Geometry check sheet. Reference: the model listing, model coordinates, mm. A direction names the side the tool comes from. Give positions to 0.01 mm unless a question says otherwise; leave off trailing zeros. Write each loop counter-clockwise with the first axis right and the second up, starting at its lowest first coordinate (ties: lowest second). Pieces come first, ordered by that corner, then holes. Notation, with made-up numbers: (57.25, 35) -> (81.25, 35) arc R7 cw to (81.25, 46) -> close; hole circle Ø7 at (-38.5, -3.75). An arc over 180 degrees is marked (long way). Write item = value, one per line. Start each with the question number.
1. Set-up check for faces 4 (the flat face through (25, 11, -15)), 5 (the flat face through (17, 23, -12)), 6 (the flat face through (3, 11, -15)), 7 (the cylindrical face through (14.07, 20.45, -12.5)): record each of +Z, -Z, +X, -X, +Y, -Y from which the full face is reachable in a straight line by a thin tool's end or side.
2. Cross-section at B-B, the plane x = 14. Record the cut outline in (y, z).
3. Cross-section at C-C, the plane z = -17. Record the cut outline in (x, y), plus the area to 3 significant figures.
4. Cross-section at A-A, the plane y = 11.5. Record the cut outline in (x, z), plus the area to 3 significant figures.
5. Thickness scan on line 1 along X through (y, z) = (19.8, -11); line 2 along Y through (x, z) = (14, -10.25); line 3 along X through (y, z) = (16.75, -1). Record the ranges inside material, lowest first.
6. Cross-section at D-D, the plane x = 8.75. Record the cut outline in (y, z), plus the area to 3 significant figures.
7. Depth check by flat-ended pin: P1, Ø10, axis at y = 8, z = -18.5, coming from the -X side; P2, Ø5, axis at y = 15, z = -13, coming from the +X side; P3, Ø1.5, axis at x = 27, y = 15, coming from the -Z side. Enter the tip coordinate at first touch or a pass-through.
8. Mould release check, pull along X, two halves, no side actions. Record for faces 1 (the cylindrical face through (12.483, 4.666, -11.339)), 2 (the flat face through (19, 6, -23)), 3 (the flat face through (0, 11, -4)): pulls with the +X half, pulls with the -X half, needs draft (parallel to the pull), parting line crosses it, or undercut.
```python
from build123d import *

# Parameters (mm, degrees)
BOSS_EXTRUDE1_DEPTH = 23
SKETCH2_R           = 7
CUT_EXTRUDE1_DEPTH  = 43.918527468
SKETCH3_R           = 1.5
CUT_EXTRUDE2_DEPTH  = 10
CHAMFER1_SIZE       = 0.5


with BuildPart() as part:
    # Sketch1 → Boss-Extrude1 (new body)
    with BuildSketch(Plane(origin=(0, 0, 0), x_dir=(1, 0, 0), z_dir=(0, 1, 0))):
        Polygon((0, 0), (28, 0), (28, 7), (25, 7), (25, 23), (3, 23), (3, 7), (0, 7), align=None)
    extrude(amount=BOSS_EXTRUDE1_DEPTH)

    # Sketch2 → Cut-Extrude1 (cut, through all)
    with BuildSketch(Plane.XY):
        with Locations((14, 11.5)):
            Circle(SKETCH2_R)
    extrude(amount=-CUT_EXTRUDE1_DEPTH, mode=Mode.SUBTRACT)

    # Sketch3 → Cut-Extrude2 (cut)
    with BuildSketch(Plane(origin=(0, 23, 0), x_dir=(1, 0, 0), z_dir=(0, 1, 0))):
        with Locations(Location((14, 11, 0), (0, 0, 270))):
            Circle(SKETCH3_R)
    extrude(amount=-CUT_EXTRUDE2_DEPTH, mode=Mode.SUBTRACT)

    # Chamfer1
    chamfer1_edges = [part.edges().sort_by_distance(p)[0] for p in [
        (14, 23, -12.5),
    ]]
    chamfer(chamfer1_edges, length=CHAMFER1_SIZE)


solid = part.part
```
Answers:
q1.face_4 = -Z, +X, +Y, -Y
q1.face_5 = +Z, -Z, +X, -X, +Y
q1.face_6 = -Z, -X, +Y, -Y
q1.face_7 = +Y
q2.outline = (0, -23) -> (4.5, -23) -> (4.5, 0) -> (0, 0) -> close; (18.5, -23) -> (23, -23) -> (23, -13) -> (22.5, -12.5) -> (18.5, -12.5) -> close; (18.5, -9.5) -> (22.5, -9.5) -> (23, -9) -> (23, 0) -> (18.5, 0) -> close
q3.outline = (3, 0) -> (25, 0) -> (25, 23) -> (3, 23) -> close; hole circle Ø14 at (14, 11.5)
q3.area = 352 mm^2
q4.outline = (0, -7) -> (3, -7) -> (3, -23) -> (7, -23) -> (7, 0) -> (0, 0) -> close; (21, -23) -> (25, -23) -> (25, -7) -> (28, -7) -> (28, 0) -> (21, 0) -> close
q4.area = 226 mm^2
q5.line_1 = 3 to 12.5, 15.5 to 25
q5.line_2 = 0 to 4.5
q5.line_3 = 0 to 9.37, 18.63 to 28
q6.outline = (0, -23) -> (6.87, -23) -> (6.87, 0) -> (0, 0) -> close; (16.13, -23) -> (23, -23) -> (23, 0) -> (16.13, 0) -> close
q6.area = 316 mm^2
q7.P1 = 3
q7.P2 = 25
q7.P3 = -7
q8.face_1 = undercut
q8.face_2 = needs draft
q8.face_3 = pulls with the -X half
